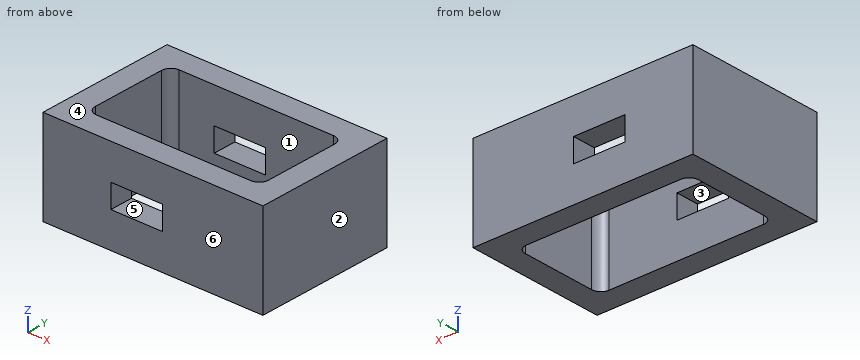
from build123d import *

# Parameters (mm, degrees)
EXTRUDE_1_DEPTH     = 20
FILLET_1_R          = 2
SKETCH_3_W          = 11
SKETCH_3_H          = 5
CUT_EXTRUDE_3_DEPTH = 31


with BuildPart() as part:
    # Sketch 1 → Extrude 1 (new body)
    with BuildSketch(Plane.XY):
        Polygon((0, 15), (-23.5, 15), (-23.5, -15), (0, -15), (0, -10), (-18.5, -10), (-18.5, 10), (0, 10), align=None)
    extrude(amount=EXTRUDE_1_DEPTH)

    # Fillet 1
    fillet_1_edges = [part.edges().sort_by_distance(p)[0] for p in [
        (-18.5, -10, 10),
        (-18.5, 10, 10),
    ]]
    fillet(fillet_1_edges, radius=FILLET_1_R)

    # Mirror 1: part across plane


with BuildPart() as part_1:
    add(part.part)
    add(part.part.mirror(Plane(origin=(0, 0, 20), x_dir=(0, 0, 1), z_dir=(1, 0, 0))))

    # Sketch 3 → Cut-Extrude 3 (cut, through all)
    with BuildSketch(Plane(origin=(0, 15, 0), x_dir=(1, 0, 0), z_dir=(0, 1, 0))):
        with Locations((-3.5, -10)):
            Rectangle(SKETCH_3_W, SKETCH_3_H)
    extrude(amount=-CUT_EXTRUDE_3_DEPTH, mode=Mode.SUBTRACT)


solid = part_1.part
Here's how the part is built. I have some questions about the finished solid (model axes, mm). Face numbers are marked on the shaded views. A direction names the side the tool comes from. Coordinates: 2 decimals unless noted, no trailing zeros. Write each loop counter-clockwise with the first axis right and the second up, starting at its lowest first coordinate (ties: lowest second). Pieces come first, ordered by that corner, then holes.
Item 1: If we mould it in two halves opening along Z, with no side actions, what happens to the marked faces 4, 5 and 6? For each: +Z half, -Z half, draft (parallel to the pull), parting line (faces both ways), or undercut.
Item 2: I want a section at B-B on y = 2.5. Write out the boundary of the cut face in (x, z).
Item 3: On a 3-axis mill with a long thin cutter (end or side, diameter ignored), from which of +Z, -Z, +X, -X, +Y, -Y can I reach the whole of each face in a straight line? I mean the marked faces 1, 2 and 3. Say none if no direction works.
Item 4: I want a section at A-A on z = 9.25. Write out the boundary of the cut face in (x, y), and give its area (3 significant figures).
Item 5: If I drill on line 1 (Y direction, x = 4, z = 10.75); line 2 (X direction, y = 2.25, z = 5.25); line 3 (Y direction, x = 17, z = 5.25), over which ranges is the centre line in solid material (lowest first)?
Item 6: I want a section at C-C on x = 12. Write out the boundary of the cut face in (y, z), and give its area (3 significant figures).
Item 7: I want a section at D-D on y = 10.75. Write out the boundary of the cut face in (x, z).
Findings below:
1. face 4: +Z half
1. face 5: undercut
1. face 6: draft
2. outline: (-23.5, 0) - (-18.5, 0) - (-18.5, 20) - (-23.5, 20) - close; (18.5, 0) - (23.5, 0) - (23.5, 20) - (18.5, 20) - close
3. face 1: +Z, -Z
3. face 2: +Z, -Z, +X, +Y, -Y
3. face 3: +Y, -Y
4. outline: (-23.5, -15) - (-9, -15) - (-9, -10) - (-16.5, -10) arc R2 cw to (-18.5, -8) - (-18.5, 8) arc R2 cw to (-16.5, 10) - (-9, 10) - (-9, 15) - (-23.5, 15) - close; (2, -15) - (23.5, -15) - (23.5, 15) - (2, 15) - (2, 10) - (16.5, 10) arc R2 cw to (18.5, 8) - (18.5, -8) arc R2 cw to (16.5, -10) - (2, -10) - close
4. area: 563 mm2
5. line 1: y = -15 to -10, 10 to 15
5. line 2: x = -23.5 to -18.5, 18.5 to 23.5
5. line 3: y = -15 to -9.94, 9.94 to 15
6. outline: (-15, 0) - (-10, 0) - (-10, 20) - (-15, 20) - close; (10, 0) - (15, 0) - (15, 20) - (10, 20) - close
6. area: 200 mm2
7. outline: (-23.5, 0) - (23.5, 0) - (23.5, 20) - (-23.5, 20) - close; hole (-9, 7.5) - (2, 7.5) - (2, 12.5) - (-9, 12.5) - close
